Model file for the job. Use its own axes, mm. Round coordinates to 2 decimals unless told otherwise and drop trailing zeros. Use a Markdown table: item, result. Add a question column.
Item 1: Pin check, flat tips, straight feed: P1, Ø3.5, axis at y = -17.5, z = -226.5, coming from the -X side; P2, Ø0.8, axis at y = 5.5, z = -190.5, coming from the -X side; P3, Ø0.5, axis at x = -5.5, z = -349.5, coming from the +Y side; P4, Ø1.5, axis at y = 4, z = -432, coming from the -X side. Stop position of each tip, or through.
Item 2: Wall check: L1, parallel to Y at x = -15, z = -107; L2, parallel to X at y = -17, z = -265.5. Give the ranges that are in metal, low to high. Write a range as from..to.
Item 3: Saw through at A-A on z = -195. Give the number of separate pieces and of enclosed holes in the cut face, then the cut area to 3 significant figures.
```python
from build123d import *

# Parameters (mm, degrees)
BOSS_EXTRU_1_DEPTH = 600


with BuildPart() as part:
    # Esquisse1 → Boss.-Extru.1 (new body)
    with BuildSketch(Plane.XY.offset(100)):
        with BuildLine():
            Line((6, -19), (6, -20))
            Line((6, -20), (17, -20))
            ThreePointArc((17, -20), (19.121320344, -19.121320344), (20, -17))
            Line((20, -17), (20, -6))
            Line((20, -6), (19, -6))
            Line((19, -6), (19, -5))
            Line((19, -5), (16, -5))
            Line((16, -5), (16, -10))
            Line((16, -10), (11.697056276, -10))
            Line((11.697056276, -10), (6.44138072, -4.744324444))
            ThreePointArc((6.44138072, -4.744324444), (7.551143817, -2.642011933), (7.994130058, -0.306405969))
            Line((7.994130058, -0.306405969), (7.7, 0))
            Line((7.7, 0), (7.994130058, 0.306405971))
            ThreePointArc((7.994130058, 0.306405971), (7.551143817, 2.642011934), (6.441380719, 4.744324444))
            Line((6.441380719, 4.744324444), (11.697056275, 10))
            Line((11.697056275, 10), (16, 10))
            Line((16, 10), (16, 5))
            Line((16, 5), (19, 5))
            Line((19, 5), (19, 6))
            Line((19, 6), (20, 6))
            Line((20, 6), (20, 17))
            ThreePointArc((20, 17), (19.121320344, 19.121320344), (17, 20))
            Line((17, 20), (6, 20))
            Line((6, 20), (6, 19))
            Line((6, 19), (5, 19))
            Line((5, 19), (5, 15.999999999))
            Line((5, 15.999999999), (10.000000001, 15.999999999))
            Line((10.000000001, 15.999999999), (10.000000001, 11.697056275))
            Line((10.000000001, 11.697056275), (4.744324444, 6.441380719))
            ThreePointArc((4.744324444, 6.441380719), (2.642011933, 7.551143817), (0.306405969, 7.994130058))
            Line((0.306405969, 7.994130058), (0, 7.7))
            Line((0, 7.7), (-0.30640597, 7.994130058))
            ThreePointArc((-0.30640597, 7.994130058), (-2.642011933, 7.551143817), (-4.744324444, 6.441380719))
            Line((-4.744324444, 6.441380719), (-9.999999999, 11.697056274))
            Line((-9.999999999, 11.697056274), (-9.999999999, 15.999999999))
            Line((-9.999999999, 15.999999999), (-5, 15.999999999))
            Line((-5, 15.999999999), (-5, 19))
            Line((-5, 19), (-6, 19))
            Line((-6, 19), (-6, 20))
            Line((-6, 20), (-17, 20))
            ThreePointArc((-17, 20), (-19.121320344, 19.121320344), (-20, 17))
            Line((-20, 17), (-20, 6))
            Line((-20, 6), (-19, 6))
            Line((-19, 6), (-19, 5))
            Line((-19, 5), (-16, 5))
            Line((-16, 5), (-16, 10))
            Line((-16, 10), (-11.697056274, 10))
            Line((-11.697056274, 10), (-6.441380718, 4.744324445))
            ThreePointArc((-6.441380718, 4.744324445), (-7.551143817, 2.642011933), (-7.994130058, 0.306405969))
            Line((-7.994130058, 0.306405969), (-7.699999999, 0))
            Line((-7.699999999, 0), (-7.994130057, -0.306405971))
            ThreePointArc((-7.994130057, -0.306405971), (-7.551143816, -2.642011934), (-6.441380719, -4.744324444))
            Line((-6.441380719, -4.744324444), (-11.697056275, -10))
            Line((-11.697056275, -10), (-16, -10))
            Line((-16, -10), (-16, -5))
            Line((-16, -5), (-19, -5))
            Line((-19, -5), (-19, -6))
            Line((-19, -6), (-20, -6))
            Line((-20, -6), (-20, -17))
            ThreePointArc((-20, -17), (-19.121320344, -19.121320344), (-17, -20))
            Line((-17, -20), (-6, -20))
            Line((-6, -20), (-6, -19))
            Line((-6, -19), (-5, -19))
            Line((-5, -19), (-5, -16.000000001))
            Line((-5, -16.000000001), (-9.999999999, -16.000000001))
            Line((-9.999999999, -16.000000001), (-9.999999999, -11.697056274))
            Line((-9.999999999, -11.697056274), (-4.744324444, -6.441380719))
            ThreePointArc((-4.744324444, -6.441380719), (-2.642011933, -7.551143817), (-0.306405969, -7.994130058))
            Line((-0.306405969, -7.994130058), (0, -7.7))
            Line((0, -7.7), (0.306405971, -7.994130058))
            ThreePointArc((0.306405971, -7.994130058), (2.642011934, -7.551143817), (4.744324445, -6.441380719))
            Line((4.744324445, -6.441380719), (10.000000001, -11.697056274))
            Line((10.000000001, -11.697056274), (10.000000001, -16.000000001))
            Line((10.000000001, -16.000000001), (5, -16.000000001))
            Line((5, -16.000000001), (5, -19))
            Line((5, -19), (6, -19))
        make_face()
        with BuildLine():
            Line((18.25, 12.25), (12.25, 12.25))
            Line((12.25, 12.25), (12.25, 18.25))
            Line((12.25, 18.25), (17.25, 18.25))
            ThreePointArc((17.25, 18.25), (17.957106781, 17.957106781), (18.25, 17.25))
            Line((18.25, 17.25), (18.25, 12.25))
        make_face(mode=Mode.SUBTRACT)
        with BuildLine():
            Line((-18.25, -12.25), (-12.25, -12.25))
            Line((-12.25, -12.25), (-12.25, -18.25))
            Line((-12.25, -18.25), (-17.25, -18.25))
            ThreePointArc((-17.25, -18.25), (-17.957106781, -17.957106781), (-18.25, -17.25))
            Line((-18.25, -17.25), (-18.25, -12.25))
        make_face(mode=Mode.SUBTRACT)
        with BuildLine():
            Line((-12.25, 18.25), (-12.25, 12.25))
            Line((-12.25, 12.25), (-18.25, 12.25))
            Line((-18.25, 12.25), (-18.25, 17.25))
            ThreePointArc((-18.25, 17.25), (-17.957106781, 17.957106781), (-17.25, 18.25))
            Line((-17.25, 18.25), (-12.25, 18.25))
        make_face(mode=Mode.SUBTRACT)
        with BuildLine():
            Line((12.25, -18.25), (12.25, -12.25))
            Line((12.25, -12.25), (18.25, -12.25))
            Line((18.25, -12.25), (18.25, -17.25))
            ThreePointArc((18.25, -17.25), (17.957106781, -17.957106781), (17.25, -18.25))
            Line((17.25, -18.25), (12.25, -18.25))
        make_face(mode=Mode.SUBTRACT)
        with BuildLine():
            Line((-5.705709703, -4.055228326), (-4.075506937, -2.896591666))
            ThreePointArc((-4.075506937, -2.896591666), (-4.635549589, -1.873947727), (-4.943520622, -0.749402378))
            Line((-4.943520622, -0.749402378), (-5.932224738, -0.899282852))
            ThreePointArc((-5.932224738, -0.899282852), (-6, 0), (-5.932224738, 0.899282853))
            Line((-5.932224738, 0.899282853), (-4.943520622, 0.749402379))
            ThreePointArc((-4.943520622, 0.749402379), (-4.635549588, 1.873947727), (-4.075506937, 2.896591666))
            Line((-4.075506937, 2.896591666), (-5.705709704, 4.055228326))
            ThreePointArc((-5.705709704, 4.055228326), (-4.953610357, 4.945881563), (-4.064132573, 5.699370705))
            Line((-4.064132573, 5.699370705), (-2.902951842, 4.070979081))
            ThreePointArc((-2.902951842, 4.070979081), (-1.877566249, 4.634085136), (-0.749402377, 4.943520623))
            Line((-0.749402377, 4.943520623), (-0.899282852, 5.932224739))
            ThreePointArc((-0.899282852, 5.932224739), (0, 6), (0.899282852, 5.932224739))
            Line((0.899282852, 5.932224739), (0.749402377, 4.943520623))
            ThreePointArc((0.749402377, 4.943520623), (1.87756625, 4.634085136), (2.902951843, 4.07097908))
            Line((2.902951843, 4.07097908), (4.064132575, 5.699370704))
            ThreePointArc((4.064132575, 5.699370704), (4.953610358, 4.945881562), (5.705709704, 4.055228326))
            Line((5.705709704, 4.055228326), (4.075506937, 2.896591666))
            ThreePointArc((4.075506937, 2.896591666), (4.635549589, 1.873947727), (4.943520623, 0.749402378))
            Line((4.943520623, 0.749402378), (5.932224739, 0.899282853))
            ThreePointArc((5.932224739, 0.899282853), (6, 0), (5.932224739, -0.899282853))
            Line((5.932224739, -0.899282853), (4.943520623, -0.749402379))
            ThreePointArc((4.943520623, -0.749402379), (4.635549589, -1.873947727), (4.075506938, -2.896591666))
            Line((4.075506938, -2.896591666), (5.705709704, -4.055228326))
            ThreePointArc((5.705709704, -4.055228326), (4.953610357, -4.945881563), (4.064132573, -5.699370705))
            Line((4.064132573, -5.699370705), (2.902951842, -4.070979081))
            ThreePointArc((2.902951842, -4.070979081), (1.87756625, -4.634085136), (0.749402378, -4.943520623))
            Line((0.749402378, -4.943520623), (0.899282852, -5.932224739))
            ThreePointArc((0.899282852, -5.932224739), (1e-09, -6), (-0.899282851, -5.932224739))
            Line((-0.899282851, -5.932224739), (-0.749402377, -4.943520623))
            ThreePointArc((-0.749402377, -4.943520623), (-1.87756625, -4.634085136), (-2.902951843, -4.07097908))
            Line((-2.902951843, -4.07097908), (-4.064132574, -5.699370704))
            ThreePointArc((-4.064132574, -5.699370704), (-4.953610357, -4.945881562), (-5.705709703, -4.055228326))
        make_face(mode=Mode.SUBTRACT)
    extrude(amount=-BOSS_EXTRU_1_DEPTH)


solid = part.part
```
Entries:
| question | item | result |
|---|---|---|
| 1 | P1 | x = -20 |
| 1 | P2 | x = -19 |
| 1 | P3 | y = 19 |
| 1 | P4 | x = -7.31 |
| 2 | L1 | -20..-18.25, -12.25..-10, 10..12.25, 18.25..20 |
| 2 | L2 | -20..-18.25, -12.25..-5, 5..12.25, 18.25..20 |
| 3 | separate pieces | 1 |
| 3 | enclosed holes | 5 |
| 3 | area | 566 mm2 |
